from build123d import *

# Parameters (mm, degrees)
EXTRUDE_1_DEPTH     = 40
SKETCH_2_W          = 25
SKETCH_2_H          = 25
EXTRUDE_2_DEPTH     = 5
SKETCH_3_W          = 20
SKETCH_3_H          = 5
CUT_EXTRUDE_1_DEPTH = 20


with BuildPart() as part:
    # 스케치1 → 보스-돌출1 (new body)
    with BuildSketch(Plane(origin=(0, 0, 0), x_dir=(1, 0, 0), z_dir=(0, 1, 0))):
        Polygon((0, 0), (25, 0), (25, 10), (10, 10), (10, 25), (0, 25), align=None)
    extrude(amount=EXTRUDE_1_DEPTH)

    # 스케치2 → 보스-돌출2 (add)
    with BuildSketch(Plane.XZ):
        with Locations((12.5, -12.5)):
            Rectangle(SKETCH_2_W, SKETCH_2_H)
    extrude(amount=EXTRUDE_2_DEPTH)

    # 스케치3 → 컷-돌출1 (cut)
    with BuildSketch(Plane(origin=(0, 0, -25), x_dir=(-1, 0, 0), z_dir=(0, 0, -1))):
        with Locations((-15, 32.5)):
            Rectangle(SKETCH_3_W, SKETCH_3_H)
    extrude(amount=-CUT_EXTRUDE_1_DEPTH, mode=Mode.SUBTRACT)


solid = part.part
Design review of the part built by this model. Coordinates are the model's own, in mm. A direction names the side the tool comes from. Round coordinates to 2 decimals unless told otherwise and drop trailing zeros. Write each loop counter-clockwise with the first axis right and the second up, starting at its lowest first coordinate (ties: lowest second). Pieces come first, ordered by that corner, then holes. Notation, with made-up numbers: (-9.75, -13) - (42.25, -13) arc R19 ccw to (42.25, 12) - close; hole circle Ø2 at (19.25, 52.25). An arc over 180 degrees is marked (long way). Return JSON: item names as keys, results as strings. Group by question number.
Item 1: The part is to be moulded in two halves that separate along Y. For faces 4 (the face through (25, 13, -7)), 5 (the face through (5, 32, -15)), 6 (the face through (12, -5, -12)), say which applies: pulls with the +Y half, pulls with the -Y half, needs draft (parallel to the pull), parting line crosses it, or undercut.
Item 2: Insertion check: P1, Ø1.5, axis at x = 17, y = 37.5, coming from the -Z side; P2, Ø2.5, axis at x = 15, y = 32.5, coming from the -Z side; P3, Ø2.5, axis at y = 36.5, z = -16, coming from the +X side. Each pin has a flat end and moves straight along its axis. Give the tip position at first contact, or say it passes through.
Item 3: We need section A-A on z = -20.25. Write out the cut boundary in (x, y), and give its area (3 significant figures).
Item 4: For probe 1 along Y at (x, z) = (22.5, -5.25); probe 2 along Y at (x, z) = (17.75, -12.5), list the stretches that pass through material, from the lowest coordinate up. Write a range as [from, to].
Item 5: We need section B-B on x = 8.5. Write out the cut boundary in (y, z).
Item 6: We need section D-D on x = 11.25. Write out the cut boundary in (y, z), and give its area (3 significant figures).
Item 7: We need section C-C on y = 8. Write out the cut boundary in (x, z), and give its area (3 significant figures).
Item 8: Machinability: for faces 1 (the face through (11, 30, -8)), 2 (the face through (10, 15, -17)), 3 (the face through (9.5, 40, -9.9)), which of the approach directions +Z, -Z, +X, -X, +Y, -Y give a long, thin tool a straight path to every point of the face, cutting with its end or side? Answer none if there is none.
Model answer:
{
 "1": {"face 4": "needs draft", "face 5": "undercut", "face 6": "pulls with the -Y half"},
 "2": {"P1": "stops at z = -10", "P2": "stops at z = -5", "P3": "stops at x = 10"},
 "3": {"outline": "(0, -5) - (25, -5) - (25, 0) - (10, 0) - (10, 30) - (5, 30) - (5, 35) - (10, 35) - (10, 40) - (0, 40) - close", "area": "500 mm²"},
 "4": {"probe 1": "y = [-5, 30], [35, 40]", "probe 2": "y = [-5, 0]"},
 "5": {"outline": "(-5, -25) - (30, -25) - (30, -5) - (35, -5) - (35, -25) - (40, -25) - (40, 0) - (-5, 0) - close"},
 "6": {"outline": "(-5, -25) - (0, -25) - (0, -10) - (30, -10) - (30, -5) - (35, -5) - (35, -10) - (40, -10) - (40, 0) - (-5, 0) - close", "area": "500 mm²"},
 "7": {"outline": "(0, -25) - (10, -25) - (10, -10) - (25, -10) - (25, 0) - (0, 0) - close", "area": "400 mm²"},
 "8": {"face 1": "-Z, +X", "face 2": "-Z, +X, +Y", "face 3": "+Z, -Z, +X, -X, +Y"}
}
